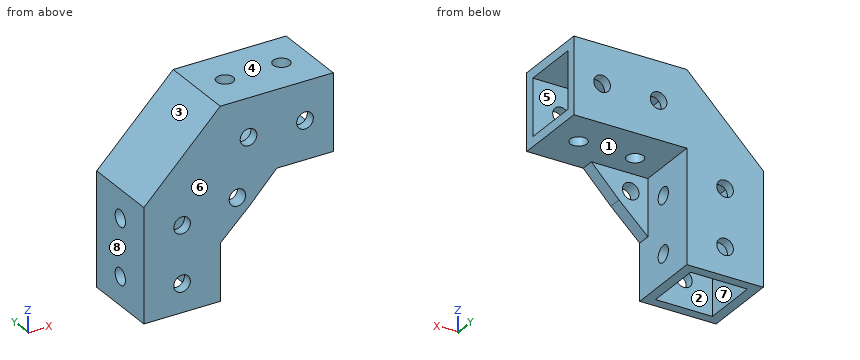
from build123d import *

# Parameters (mm, degrees)
SKETCH1_W           = 34
SKETCH1_H           = 23
SKETCH1_R           = 2.5
BOSS_EXTRUDE1_DEPTH = 23
SKETCH6_OUTSIDE_W   = 45.41
SKETCH6_OUTSIDE_H   = 34.41
SKETCH6_OUTSIDE_W_2 = 34
SKETCH6_OUTSIDE_H_2 = 23
SKETCH6_OUTSIDE_R   = 2.5
CUT_EXTRUDE10_DEPTH = 24
SKETCH7_OUTSIDE_W   = 34.41
SKETCH7_OUTSIDE_H   = 34.41
SKETCH7_OUTSIDE_W_2 = 23
SKETCH7_OUTSIDE_H_2 = 23
SKETCH7_OUTSIDE_W_3 = 17.12
SKETCH7_OUTSIDE_H_3 = 17.12
CUT_EXTRUDE11_DEPTH = 34
BOSS_EXTRUDE2_DEPTH = 23
SKETCH13_R          = 2.5
BOSS_EXTRUDE3_DEPTH = 4


with BuildPart() as part:
    # sketch1 → Boss-Extrude1 (new body)
    with BuildSketch(Plane(origin=(0, 0, 0), x_dir=(1, 0, 0), z_dir=(0, 1, 0))):
        with Locations((17, -11.5)):
            Rectangle(SKETCH1_W, SKETCH1_H)
        with Locations((8.5, -11.5)):
            Circle(SKETCH1_R, mode=Mode.SUBTRACT)
        with Locations((25.5, -11.5)):
            Circle(SKETCH1_R, mode=Mode.SUBTRACT)
    extrude(amount=BOSS_EXTRUDE1_DEPTH)

    # Sketch6 outside → Cut-Extrude10 (cut, through all)
    with BuildSketch(Plane(origin=(0, 0, 0), x_dir=(-1, 0, 0), z_dir=(0, 0, -1))):
        with Locations((-17, 11.5)):
            Rectangle(SKETCH6_OUTSIDE_W, SKETCH6_OUTSIDE_H)
        with Locations((-17, 11.5)):
            Rectangle(SKETCH6_OUTSIDE_W_2, SKETCH6_OUTSIDE_H_2, mode=Mode.SUBTRACT)
        with Locations((-25.5, 11.5)):
            Circle(SKETCH6_OUTSIDE_R)
        with Locations((-8.5, 11.5)):
            Circle(SKETCH6_OUTSIDE_R)
    extrude(amount=-CUT_EXTRUDE10_DEPTH, mode=Mode.SUBTRACT)

    # Sketch7 outside → Cut-Extrude11 (cut)
    with BuildSketch(Plane(origin=(34, 0, 0), x_dir=(0, 0, -1), z_dir=(1, 0, 0))):
        with Locations((-11.5, 11.5)):
            Rectangle(SKETCH7_OUTSIDE_W, SKETCH7_OUTSIDE_H)
        with Locations((-11.5, 11.5)):
            Rectangle(SKETCH7_OUTSIDE_W_2, SKETCH7_OUTSIDE_H_2, mode=Mode.SUBTRACT)
        with Locations((-11.5, 11.5)):
            Rectangle(SKETCH7_OUTSIDE_W_3, SKETCH7_OUTSIDE_H_3)
    extrude(amount=-CUT_EXTRUDE11_DEPTH, mode=Mode.SUBTRACT)


with BuildPart() as body_2:
    # Mirror6: mirrored copy
    add(part.part.mirror(Plane(origin=(0, 0, 0), x_dir=(-0.707106781, 0, 0.707106781), z_dir=(-0.707106781, 0, -0.707106781))))


with BuildPart() as part_1:
    add(part.part)

    add(body_2.part)  # Boss-Extrude2 merges body 2
    # Sketch11 → Boss-Extrude2 (add)
    with BuildSketch(Plane(origin=(0, 0, 0), x_dir=(1, 0, 0), z_dir=(0, 1, 0))):
        Polygon((-23, 0), (0, -23), (0, 0), align=None)
    extrude(amount=BOSS_EXTRUDE2_DEPTH)

    # Sketch13 → Boss-Extrude3 (add)
    with BuildSketch(Plane(origin=(0, 0, 0), x_dir=(1, 0, 0), z_dir=(0, 1, 0))):
        Polygon((8.706365938, 8.706365938), (0, 17), (0, 0), (17, 0), align=None)
        with Locations((5.170832032, 5.170832032)):
            Circle(SKETCH13_R, mode=Mode.SUBTRACT)
    extrude(amount=BOSS_EXTRUDE3_DEPTH)


solid = part_1.part
Source: CAD feature listing. Evaluate the final solid. Frame: model axes, mm. Face numbers are marked on the shaded views. A direction names the side the tool comes from. Round coordinates to 2 decimals unless told otherwise and drop trailing zeros. Loops run counter-clockwise (first coordinate to the right, second up) from the corner with the lowest first, then second, coordinate; pieces in that order, holes last.
Q1. First-contact query: P1, Ø2, axis at x = 18, y = 5, coming from the -Z side; P2, Ø13.5, axis at y = 12, z = -11.5, coming from the +X side; P3, Ø8, axis at x = -6, y = 12.5, coming from the +Z side. Flat tips, straight axial feed; report the tip coordinate or a pass-through.
Q2. Section B-B, the plane z = 11.5. Return loops of the section in (x, y), plus the area to 3 significant figures.
Q3. Section A-A, the plane x = -11.5. Return loops of the section in (y, z).
Q4. Access query for the marked faces 1, 2, 3, 4 and 5. Directions: +Z, -Z, +X, -X, +Y, -Y. A direction counts if a zero-diameter tool reaches every point of the face in a straight line with its end or side. Return the directions, or none.
Q5. Ray query, line 1 (X direction, y = 4, z = -26); line 2 (Z direction, x = 12.5, y = 10.75); line 3 (Y direction, x = -1.05, z = -8.5). Return the intervals inside material, ascending.
Q6. Mould query, pull axis Y, two halves, no side actions, for the marked faces 6, 7 and 8. Classes: pulls with the +Y half, pulls with the -Y half, needs draft (parallel to the pull), parting line crosses it, or undercut.
Q7. Section C-C, the plane x = 4. Return loops of the section in (y, z).
Q8. Section D-D, the plane z = -25.5. Return loops of the section in (x, y).
Solutions:
1. P1: stops at z = 0
1. P2: stops at x = 0
1. P3: stops at z = 21
2. outline: (-11.5, 0) - (6, 0) - (6, 2.94) - (0, 2.94) - (0, 20.06) - (6, 20.06) - (6, 23) - (-11.5, 23) - close; (11, 0) - (23, 0) - (23, 2.94) - (11, 2.94) - close; (11, 20.06) - (23, 20.06) - (23, 23) - (11, 23) - close; (28, 0) - (34, 0) - (34, 2.94) - (28, 2.94) - close; (28, 20.06) - (34, 20.06) - (34, 23) - (28, 23) - close
2. area: 406 mm2
3. outline: (0, -34) - (2.94, -34) - (2.94, -28) - (0, -28) - close; (0, -23) - (2.94, -23) - (2.94, -11) - (0, -11) - close; (0, -6) - (2.94, -6) - (2.94, 0) - (20.06, 0) - (20.06, -6) - (23, -6) - (23, 11.5) - (0, 11.5) - close; (20.06, -34) - (23, -34) - (23, -28) - (20.06, -28) - close; (20.06, -23) - (23, -23) - (23, -11) - (20.06, -11) - close
4. face 1: -Z, +X, +Y
4. face 2: -Z
4. face 3: +Z, -X, +Y, -Y
4. face 4: +Z, +X, -X, +Y, -Y
4. face 5: +X
5. line 1: x = -23 to -20.06, -2.94 to 0
5. line 2: z = 0 to 2.94, 20.06 to 23
5. line 3: y = 0 to 9, 14 to 23
6. face 6: pulls with the -Y half
6. face 7: undercut
6. face 8: needs draft
7. outline: (0, -13.19) - (4, -13.19) - (4, -7.38) - (0, -7.38) - close; (0, -2.96) - (4, -2.96) - (4, 0) - (23, 0) - (23, 23) - (0, 23) - close; hole (2.94, 2.94) - (20.06, 2.94) - (20.06, 20.06) - (2.94, 20.06) - close
8. outline: (-23, 0) - (-14, 0) - (-14, 2.94) - (-20.06, 2.94) - (-20.06, 9) - (-23, 9) - close; (-23, 14) - (-20.06, 14) - (-20.06, 20.06) - (-14, 20.06) - (-14, 23) - (-23, 23) - close; (-9, 0) - (0, 0) - (0, 9) - (-2.94, 9) - (-2.94, 2.94) - (-9, 2.94) - close; (-9, 20.06) - (-2.94, 20.06) - (-2.94, 14) - (0, 14) - (0, 23) - (-9, 23) - close
